Input: part model. Units: mm. Frame: model coordinates. Face numbers are marked on the shaded views. A direction names the side the tool comes from. Coordinates: 2 decimals unless noted, no trailing zeros. Order: outer loops, then holes, each group sorted by start corner. A loop starts at its lowest first (then second) coordinate and runs counter-clockwise, first axis right, second up. Notation, with made-up numbers: (29, 67.5) -> (43, 67.5) arc R13 ccw to (43, 76.5) -> close; hole circle Ø9 at (-0.5, 32.25). An arc over 180 degrees is marked (long way). Answer as CSV lines item,"result".
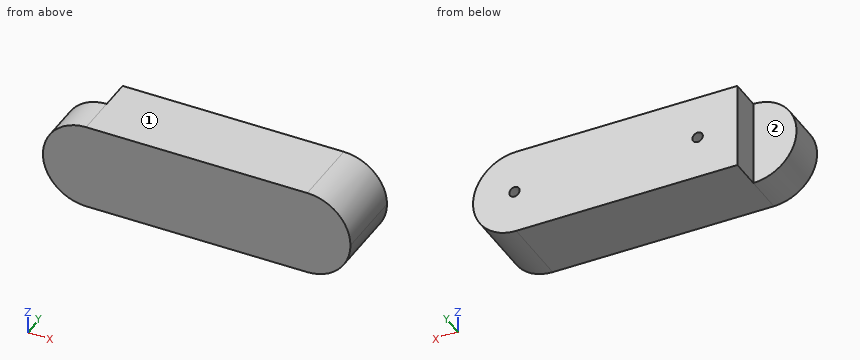
from build123d import *

# Parameters (mm, degrees)
BOSS_EXTRUDE1_DEPTH = 20.6
CUT_EXTRUDE1_START  = -9
CUT_EXTRUDE1_DEPTH  = 9
SKETCH4_R           = 1.5
CUT_EXTRUDE2_DEPTH  = 4


with BuildPart() as part:
    # Sketch1 → Boss-Extrude1 (new body)
    with BuildSketch(Plane(origin=(0, 0, 0), x_dir=(1, 0, 0), z_dir=(0, 1, 0))):
        with BuildLine():
            ThreePointArc((0, 25), (-12.5, 12.5), (0, 0))
            Line((0, 0), (0, 25))
        make_face()
        with BuildLine():
            Line((0, 25), (0, 0))
            ThreePointArc((0, 0), (8.838834765, 3.661165235), (12.5, 12.5))
            ThreePointArc((12.5, 12.5), (8.838834765, 21.338834765), (0, 25))
        make_face()
        with BuildLine():
            ThreePointArc((12.5, 12.5), (8.838834765, 3.661165235), (0, 0))
            Line((0, 0), (64, 0))
            ThreePointArc((64, 0), (51.5, 12.5), (64, 25))
            Line((64, 25), (0, 25))
            ThreePointArc((0, 25), (8.838834765, 21.338834765), (12.5, 12.5))
        make_face()
        with BuildLine():
            ThreePointArc((64, 25), (51.5, 12.5), (64, 0))
            Line((64, 0), (64, 25))
        make_face()
        with BuildLine():
            Line((64, 25), (64, 0))
            ThreePointArc((64, 0), (72.838834765, 3.661165235), (76.5, 12.5))
            ThreePointArc((76.5, 12.5), (72.838834765, 21.338834765), (64, 25))
        make_face()
    extrude(amount=BOSS_EXTRUDE1_DEPTH)

    # Sketch3 → Cut-Extrude1 (cut)
    with BuildSketch(Plane(origin=(0, 20.6, 0), x_dir=(1, 0, 0), z_dir=(0, 1, 0)).offset(CUT_EXTRUDE1_START)):
        with BuildLine():
            Line((0, 0), (0, 25))
            ThreePointArc((0, 25), (-12.5, 12.5), (0, 0))
        make_face()
    extrude(amount=CUT_EXTRUDE1_DEPTH, mode=Mode.SUBTRACT)

    # Sketch4 → Cut-Extrude2 (cut)
    with BuildSketch(Plane(origin=(0, 20.6, 0), x_dir=(1, 0, 0), z_dir=(0, 1, 0))):
        with Locations(Location((64.5, 12.5, 0), (0, 0, 270))):
            Circle(SKETCH4_R)
        with Locations(Location((11.5, 12.5, 0), (0, 0, 270))):
            Circle(SKETCH4_R)
    extrude(amount=-CUT_EXTRUDE2_DEPTH, mode=Mode.SUBTRACT)


solid = part.part
1. Cut plane D-D (z = -18.25). Return the cut outline in (x, y), plus the area to 3 significant figures.
Findings:
outline,"(-11.1, 0) -> (75.1, 0) -> (75.1, 20.6) -> (0, 20.6) -> (0, 11.6) -> (-11.1, 11.6) -> close"
area,"1,680 mm2"
2. Ray query, line 1 along X through (y, z) = (18.95, -12.5); line 2 along Z through (x, y) = (64.5, 17.75); line 3 along X through (y, z) = (17, -13.75). Return the intervals inside material, ascending.
Findings:
line 1,"x = 0 to 10, 13 to 63, 66 to 76.5"
line 2,"z = -24.99 to -14, -11 to -0.01"
line 3,"x = 0 to 10.67, 12.33 to 63.67, 65.33 to 76.44"
3. Cut plane A-A (y = 18). Return the cut outline in (x, z).
Findings:
outline,"(0, -25) -> (64, -25) arc R12.5 ccw to (64, 0) -> (0, 0) -> close; hole circle Ø3 at (11.5, -12.5); hole circle Ø3 at (64.5, -12.5)"
4. Contact query for flat-ended pins moving along their axis: pin 1 (10 mm diameter, centred on x = -1.5, y = 2.5, fed in from -Z); pin 2 (1.5 mm diameter, centred on x = 64.5, z = -12, fed in from +Y); pin 3 (10 mm diameter, centred on y = 3, z = -19.5, fed in from -X); pin 4 (7 mm diameter, centred on y = 16.5, z = -13.5, fed in from -X). Output: stop coordinate, or through.
Findings:
pin 1,"stops at z = -25"
pin 2,"stops at y = 16.6"
pin 3,"stops at x = -12.34"
pin 4,"stops at x = 0"
5. Cut plane B-B (x = 11.5). Return the cut outline in (y, z), plus the area to 3 significant figures.
Findings:
outline,"(0, -25) -> (20.6, -25) -> (20.6, -14) -> (16.6, -14) -> (16.6, -11) -> (20.6, -11) -> (20.6, 0) -> (0, 0) -> close"
area,"503 mm2"
6. Reachability of the marked faces 1 and 2 from +Z, -Z, +X, -X, +Y, -Y: full face, straight path, thin tool, end or side. Return the list, or none.
Findings:
face 1,"+Z, +X, -X, +Y, -Y"
face 2,"+Z, -Z, -X, +Y"
7. Cut plane C-C (y = 4). Return the cut outline in (x, z), plus the area to 3 significant figures.
Findings:
outline,"(0, -25) -> (64, -25) arc R12.5 ccw to (64, 0) -> (0, 0) arc R12.5 ccw to start"
area,"2,090 mm2"
